Geometry check sheet. Reference: the model listing, model coordinates, mm. A direction names the side the tool comes from. Round coordinates to 2 decimals unless told otherwise and drop trailing zeros. Loops run counter-clockwise (first coordinate to the right, second up) from the corner with the lowest first, then second, coordinate; pieces in that order, holes last. Notation, with made-up numbers: (35, 19.5) -> (79, 19.5) arc R20 cw to (79, 25.5) -> close; hole circle Ø2 at (73, 30.25). An arc over 180 degrees is marked (long way). Use one line per item in the form item = value.
from build123d import *

# Parameters (mm, degrees)
SKETCH1_W                = 100
SKETCH1_H                = 100
BOSS_EXTRUDE1_DEPTH      = 1.5
CUT_EXTRUDE6_DEPTH       = 71.774289117
SKETCH4_W                = 27.5
SKETCH4_H                = 3.18
CUT_EXTRUDE9_DEPTH       = 3
CUT_EXTRUDE10_DEPTH      = 3
MIRROR10_COPY_1_SKETCH_W = 27.5
MIRROR10_COPY_1_SKETCH_H = 3.18
MIRROR10_COPY_1_DEPTH    = 3
SKETCH27_W               = 18.2
SKETCH27_H               = 3.2
CUT_EXTRUDE19_DEPTH      = 3
SKETCH38_W               = 12.6
SKETCH38_H               = 13.5
BOSS_EXTRUDE5_DEPTH      = 3
SKETCH39_W               = 12.5
SKETCH39_H               = 13.6
CUT_EXTRUDE30_DEPTH      = 3


with BuildPart() as part:
    # Sketch1 → Boss-Extrude1 (new, symmetric)
    with BuildSketch(Plane(origin=(0, 0, 0), x_dir=(1, 0, 0), z_dir=(0, 1, 0))):
        Rectangle(SKETCH1_W, SKETCH1_H)
    extrude(amount=BOSS_EXTRUDE1_DEPTH, both=True)

    # Sketch2 → Cut-Extrude6 (cut, through all)
    with BuildSketch(Plane(origin=(0, 1.5, 0), x_dir=(1, 0, 0), z_dir=(0, 1, 0))):
        Polygon((-7.5, -50), (-7.5, -46.82), (-1.47, -46.82), (-1.47, -39.02), (-3.25, -39.02), (-3.25, -36.42), (-1.47, -36.42), (-1.47, -30.8), (1.47, -30.8), (1.47, -36.42), (3.25, -36.42), (3.25, -39.02), (1.47, -39.02), (1.47, -46.82), (7.5, -46.82), (7.5, -50), align=None)
    cut_extrude6 = extrude(amount=-CUT_EXTRUDE6_DEPTH, mode=Mode.SUBTRACT)

    # Mirror1: Cut-Extrude6 across plane
    add(cut_extrude6.mirror(Plane.XY), mode=Mode.SUBTRACT)

    # Sketch4 → Cut-Extrude9 (cut)
    with BuildSketch(Plane(origin=(0, 1.5, 0), x_dir=(1, 0, 0), z_dir=(0, 1, 0))):
        with Locations((-36.25, 48.41)):
            Rectangle(SKETCH4_W, SKETCH4_H)
    cut_extrude9 = extrude(amount=-CUT_EXTRUDE9_DEPTH, mode=Mode.SUBTRACT)

    # Sketch5 → Cut-Extrude10 (cut)
    with BuildSketch(Plane.XZ.offset(1.5)):
        Polygon((50, -7.5), (50, 7.5), (46.82, 7.5), (46.82, 1.47), (39.02, 1.47), (39.02, 3.25), (36.42, 3.25), (36.42, 1.47), (30.8, 1.47), (30.8, -1.47), (36.42, -1.47), (36.42, -3.25), (39.02, -3.25), (39.02, -1.47), (46.82, -1.47), (46.82, -7.5), align=None)
    cut_extrude10 = extrude(amount=-CUT_EXTRUDE10_DEPTH, mode=Mode.SUBTRACT)

    # Mirror6: Cut-Extrude10 across plane
    add(cut_extrude10.mirror(Plane(origin=(0, 0, 0), x_dir=(0, 0, 1), z_dir=(1, 0, 0))), mode=Mode.SUBTRACT)

    # Mirror9: Cut-Extrude9 across plane
    add(cut_extrude9.mirror(Plane.XY), mode=Mode.SUBTRACT)

    # Mirror10: Cut-Extrude9 across plane
    add(cut_extrude9.mirror(Plane(origin=(0, 0, 0), x_dir=(0, 0, 1), z_dir=(1, 0, 0))), mode=Mode.SUBTRACT)

    # Mirror10 copy 1 sketch → Mirror10 copy 1 (cut)
    with BuildSketch(Plane(origin=(0, 1.5, 0), x_dir=(-1, 0, 0), z_dir=(0, 1, 0))):
        with Locations((-36.25, 48.41)):
            Rectangle(MIRROR10_COPY_1_SKETCH_W, MIRROR10_COPY_1_SKETCH_H)
    extrude(amount=-MIRROR10_COPY_1_DEPTH, mode=Mode.SUBTRACT)

    # Sketch27 → Cut-Extrude19 (cut)
    with BuildSketch(Plane.XZ.offset(1.5)):
        with Locations((-25.9, 20.22)):
            Rectangle(SKETCH27_W, SKETCH27_H)
    extrude(amount=-CUT_EXTRUDE19_DEPTH, mode=Mode.SUBTRACT)

    # Sketch38 → Boss-Extrude5 (add)
    with BuildSketch(Plane(origin=(0, 1.5, 0), x_dir=(1, 0, 0), z_dir=(0, 1, 0))):
        with Locations((40.4, -19.07)):
            Rectangle(SKETCH38_W, SKETCH38_H)
    extrude(amount=-BOSS_EXTRUDE5_DEPTH)

    # Sketch39 → Cut-Extrude30 (cut)
    with BuildSketch(Plane(origin=(0, 1.5, 0), x_dir=(1, 0, 0), z_dir=(0, 1, 0))):
        with Locations((39.35, -19.02)):
            Rectangle(SKETCH39_W, SKETCH39_H)
    extrude(amount=-CUT_EXTRUDE30_DEPTH, mode=Mode.SUBTRACT)


solid = part.part
1. Section check B-B (x = -25.5). Record the boundary of the cut face in (y, z), then the cut area to 3 significant figures.
Return value:
outline = (-1.5, -46.82) -> (1.5, -46.82) -> (1.5, 18.62) -> (-1.5, 18.62) -> close; (-1.5, 21.82) -> (1.5, 21.82) -> (1.5, 46.82) -> (-1.5, 46.82) -> close
area = 271 mm2
2. Mould release check, pull along Z, two halves, no side actions. Record for faces 1 (the flat face through (4, 0, -46.82)), 2 (the flat face through (-26, 0, 21.82)), 3 (the flat face through (-1, -1.5, -1)): released by +Z, released by -Z, zero draft, split by the parting line, or undercut.
Return value:
face_1 = released by -Z
face_2 = undercut
face_3 = zero draft
3. Section check A-A (z = 16). Record the boundary of the cut face in (x, y).
Return value:
outline = (-50, -1.5) -> (33.1, -1.5) -> (33.1, 1.5) -> (-50, 1.5) -> close; (45.6, -1.5) -> (50, -1.5) -> (50, 1.5) -> (45.6, 1.5) -> close
4. Gauge pin test, flat ends, axial feed: pin 1 (0.9 mm diameter, centred on y = 0.5, z = -48.5, fed in from +X); pin 2 (1.4 mm diameter, centred on x = 2, y = 0, fed in from -Z); pin 3 (1.4 mm diameter, centred on y = 0, z = 2, fed in from +X). Record the tip position at first contact, or that the pin passes through.
Return value:
pin_1 = 22.5
pin_2 = -46.82
pin_3 = 46.82
5. Section check C-C (y = -0.25). Count the separate pieces of the cut face and the enclosed holes in it, then the cut area to 3 significant figures.
Return value:
separate_pieces = 1
enclosed_holes = 2
area = 9,010 mm2
6. Material ranges on line 1 along X through (y, z) = (1.3, 2.5); line 2 along Z through (x, y) = (-34.5, 0); line 3 along X through (y, z) = (-1.3, -42.5), recorded low to high.
Return value:
line_1 = -46.82 to -39.02, -36.42 to 36.42, 39.02 to 46.82
line_2 = -46.82 to -1.47, 1.47 to 18.62, 21.82 to 46.82
line_3 = -50 to -1.47, 1.47 to 50
7. Tool access check on faces 4 (the flat face through (39, 0, 12.22)), 5 (the flat face through (22.5, 0, 48)), 6 (the flat face through (22.5, 0, -48)), 7 (the flat face through (-22.5, 0, -48)), 8 (the flat face through (46.82, 0, 5)). Record the directions out of +Z, -Z, +X, -X, +Y, -Y that give a thin tool (end or side, any length) a straight path to the whole face; none if there is none.
Return value:
face_4 = +Y, -Y
face_5 = +Z, +X, +Y, -Y
face_6 = -Z, +X, +Y, -Y
face_7 = -Z, -X, +Y, -Y
face_8 = +X, +Y, -Y
